Work out the finished part from the listing and answer in its coordinate system (mm). A direction names the side the tool comes from. Coordinates: 2 decimals unless noted, no trailing zeros. Write each loop counter-clockwise with the first axis right and the second up, starting at its lowest first coordinate (ties: lowest second). Pieces come first, ordered by that corner, then holes. Notation, with made-up numbers: (-21.75, -15.5) - (3.25, -15.5) arc R15 ccw to (3.25, 7.5) - close; hole circle Ø6 at (-15.75, 73). An arc over 180 degrees is marked (long way). Use a Markdown table: item, result. Add a question column.
(1) Find the intervals of material crossed by line 1 (Y direction, x = -85, z = 13.75); line 2 (X direction, y = 124, z = 3.5); line 3 (Y direction, x = -81.5, z = 11.5), in increasing order. Write a range as from..to.
(2) The part is cut by section B-B, the plane z = 8.75. Give the vertices of the cut face in (x, y).
(3) Given pin 1 Ø6 at (y, z) = (8, 9) entering from +X; pin 2 Ø1.5 at (x, z) = (70.5, 2) entering from +Y; pin 3 Ø1 at (x, z) = (91, 3.5) entering from +Y, each flat-ended and moving along its own axis, determine where each tip first touches the part or whether it passes through.
(4) The part is cut by section A-A, the plane y = 130. Give the vertices of the cut face in (x, z), then the cut area to 3 significant figures.
(5) For a pull along Y with two mould halves and no side action, classify faces 6 (the face through (75, -104.5, 8)), 7 (the face through (61.8, -53, 7.4)), 8 (the face through (-30, -225, 7)), 9 (the face through (57, -112, 8)) as released by +Y, released by -Y, zero draft, split by the parting line, or undercut.
(6) A tool of negligible diameter and unlimited length cuts with its end or side. For faces 1 (the face through (-30, 127, 7)), 2 (the face through (80, -120, 8)), 3 (the face through (89, -200, 7)), 4 (the face through (-75, -104.5, 8)), 5 (the face through (-1.63, 42.68, 7.4)), from which of +Z, -Z, +X, -X, +Y, -Y can it reach the whole face along a straight path? Write none if from no direction.
(7) The part is cut by section D-D, the plane y = -130. Give the vertices of the cut face in (x, z).
(8) The part is cut by section C-C, the plane x = -64. Give the vertices of the cut face in (y, z).
from build123d import *

# Parameters (mm, degrees)
ESQUISSE1_R             = 7.5
BOSS_EXTRU_1_DEPTH      = 15
ESQUISSE2_W             = 90.989913166
ESQUISSE2_H             = 15.5
ENL_V_MAT_EXTRU_1_DEPTH = 15


with BuildPart() as part:
    # Esquisse1 → Boss.-Extru.1 (new body)
    with BuildSketch(Plane.XY):
        Polygon((-30, 0), (-150, -200), (-30, -200), (-30, -250), (30, -250), (30, -200), (150, -200), (30, 0), (30, 250), (-30, 250), align=None)
        with Locations((0, 210)):
            Circle(ESQUISSE1_R, mode=Mode.SUBTRACT)
        with Locations((0, 170)):
            Circle(ESQUISSE1_R, mode=Mode.SUBTRACT)
        with Locations((0, 130)):
            Circle(ESQUISSE1_R, mode=Mode.SUBTRACT)
        with Locations((0, 90)):
            Circle(ESQUISSE1_R, mode=Mode.SUBTRACT)
        with Locations((0, 50)):
            Circle(ESQUISSE1_R, mode=Mode.SUBTRACT)
        with Locations((0, 10)):
            Circle(ESQUISSE1_R, mode=Mode.SUBTRACT)
    extrude(amount=BOSS_EXTRU_1_DEPTH)

    # Esquisse2 → Enlèv. mat.-Extru.1 (cut)
    with BuildSketch(Plane.XY.offset(15)):
        with Locations((-102.494956583, -112.25)):
            Rectangle(ESQUISSE2_W, ESQUISSE2_H)
    enl_v_mat_extru_1 = extrude(amount=-ENL_V_MAT_EXTRU_1_DEPTH, mode=Mode.SUBTRACT)

    # Symétrie1: Enlèv. mat.-Extru.1 across plane
    add(enl_v_mat_extru_1.mirror(Plane(origin=(0, 0, 0), x_dir=(0, 0, 1), z_dir=(1, 0, 0))), mode=Mode.SUBTRACT)


solid = part.part
Model answer:
| question | item | result |
|---|---|---|
| 1 | line 1 | -200..-120, -104.5..-91.67 |
| 1 | line 2 | -30..-4.5, 4.5..30 |
| 1 | line 3 | -200..-120, -104.5..-85.83 |
| 2 | outline | (-150, -200) - (-30, -200) - (-30, -250) - (30, -250) - (30, -200) - (150, -200) - (102, -120) - (57, -120) - (57, -104.5) - (92.7, -104.5) - (30, 0) - (30, 250) - (-30, 250) - (-30, 0) - (-92.7, -104.5) - (-57, -104.5) - (-57, -120) - (-102, -120) - close; hole circle Ø15 at (0, 10); hole circle Ø15 at (0, 50); hole circle Ø15 at (0, 90); hole circle Ø15 at (0, 130); hole circle Ø15 at (0, 170); hole circle Ø15 at (0, 210) |
| 3 | pin 1 | x = 30 |
| 3 | pin 2 | y = -66.25 |
| 3 | pin 3 | y = -100.83 |
| 4 | outline | (-30, 0) - (-7.5, 0) - (-7.5, 15) - (-30, 15) - close; (7.5, 0) - (30, 0) - (30, 15) - (7.5, 15) - close |
| 4 | area | 675 mm^2 |
| 5 | face 6 | undercut |
| 5 | face 7 | released by +Y |
| 5 | face 8 | zero draft |
| 5 | face 9 | undercut |
| 6 | face 1 | +Z, -Z, -X, +Y |
| 6 | face 2 | +Z, -Z, +X |
| 6 | face 3 | +Z, -Z, +X, -Y |
| 6 | face 4 | +Z, -Z, -X |
| 6 | face 5 | +Z, -Z |
| 7 | outline | (-108, 0) - (108, 0) - (108, 15) - (-108, 15) - close |
| 8 | outline | (-200, 0) - (-120, 0) - (-120, 15) - (-200, 15) - close; (-104.5, 0) - (-56.67, 0) - (-56.67, 15) - (-104.5, 15) - close |
